Input: part model. Units: mm. Frame: model coordinates. A direction names the side the tool comes from. Round coordinates to 2 decimals unless told otherwise and drop trailing zeros. Loops run counter-clockwise (first coordinate to the right, second up) from the corner with the lowest first, then second, coordinate; pieces in that order, holes last. Notation, with made-up numbers: (55.5, 77) -> (61.5, 77) arc R33 ccw to (61.5, 107) -> close; hole circle Ø7 at (34.5, -5). An arc over 180 degrees is marked (long way). Answer as a JSON object with one key per item and string values.
```python
from build123d import *

# Parameters (mm, degrees)
SKETCH1_R           = 8.8
SKETCH1_R_2         = 3
BOSS_EXTRUDE1_DEPTH = 19.5
SKETCH2_OUTSIDE_W   = 25.924
SKETCH2_OUTSIDE_H   = 25.924
SKETCH2_OUTSIDE_R   = 4.5
CUT_EXTRUDE1_DEPTH  = 6.5
SKETCH3_OUTSIDE_W   = 25.924
SKETCH3_OUTSIDE_H   = 25.924
SKETCH3_OUTSIDE_R   = 6.8
CUT_EXTRUDE2_DEPTH  = 11
SKETCH5_OUTSIDE_W   = 25.924
SKETCH5_OUTSIDE_H   = 25.924
SKETCH5_OUTSIDE_R   = 4.8
CUT_EXTRUDE3_DEPTH  = 7.5
CUT_EXTRUDE4_START  = -1
SKETCH4_OUTSIDE_W   = 25.924
SKETCH4_OUTSIDE_H   = 25.924
SKETCH4_OUTSIDE_R   = 6
CUT_EXTRUDE4_DEPTH  = 1
CUT_EXTRUDE5_START  = -1
SKETCH6_OUTSIDE_W   = 25.924
SKETCH6_OUTSIDE_H   = 25.924
SKETCH6_OUTSIDE_R   = 4
CUT_EXTRUDE5_DEPTH  = 1
CUT_EXTRUDE6_START  = -3
SKETCH6_2_OUTSIDE_W = 25.924
SKETCH6_2_OUTSIDE_H = 25.924
SKETCH6_2_OUTSIDE_R = 4
CUT_EXTRUDE6_DEPTH  = 2
CHAMFER1_SIZE       = 0.5


with BuildPart() as part:
    # Sketch1 → Boss-Extrude1 (new body)
    with BuildSketch(Plane.XY):
        Circle(SKETCH1_R)
        Circle(SKETCH1_R_2, mode=Mode.SUBTRACT)
    extrude(amount=BOSS_EXTRUDE1_DEPTH)

    # Sketch2 outside → Cut-Extrude1 (cut)
    with BuildSketch(Plane.XY.offset(19.5)):
        Rectangle(SKETCH2_OUTSIDE_W, SKETCH2_OUTSIDE_H)
        Circle(SKETCH2_OUTSIDE_R, mode=Mode.SUBTRACT)
    extrude(amount=-CUT_EXTRUDE1_DEPTH, mode=Mode.SUBTRACT)

    # Sketch3 outside → Cut-Extrude2 (cut)
    with BuildSketch(Plane(origin=(0, 0, 0), x_dir=(-1, 0, 0), z_dir=(0, 0, -1))):
        Rectangle(SKETCH3_OUTSIDE_W, SKETCH3_OUTSIDE_H)
        Circle(SKETCH3_OUTSIDE_R, mode=Mode.SUBTRACT)
    extrude(amount=-CUT_EXTRUDE2_DEPTH, mode=Mode.SUBTRACT)

    # Sketch5 outside → Cut-Extrude3 (cut)
    with BuildSketch(Plane(origin=(0, 0, 0), x_dir=(-1, 0, 0), z_dir=(0, 0, -1))):
        Rectangle(SKETCH5_OUTSIDE_W, SKETCH5_OUTSIDE_H)
        Circle(SKETCH5_OUTSIDE_R, mode=Mode.SUBTRACT)
    extrude(amount=-CUT_EXTRUDE3_DEPTH, mode=Mode.SUBTRACT)

    # Sketch4 outside → Cut-Extrude4 (cut)
    with BuildSketch(Plane(origin=(0, 0, 7.5), x_dir=(-1, 0, 0), z_dir=(0, 0, -1)).offset(CUT_EXTRUDE4_START)):
        Rectangle(SKETCH4_OUTSIDE_W, SKETCH4_OUTSIDE_H)
        Circle(SKETCH4_OUTSIDE_R, mode=Mode.SUBTRACT)
    extrude(amount=-CUT_EXTRUDE4_DEPTH, mode=Mode.SUBTRACT)

    # Sketch6 outside → Cut-Extrude5 (cut)
    with BuildSketch(Plane(origin=(0, 0, 0), x_dir=(-1, 0, 0), z_dir=(0, 0, -1)).offset(CUT_EXTRUDE5_START)):
        Rectangle(SKETCH6_OUTSIDE_W, SKETCH6_OUTSIDE_H)
        Circle(SKETCH6_OUTSIDE_R, mode=Mode.SUBTRACT)
    extrude(amount=-CUT_EXTRUDE5_DEPTH, mode=Mode.SUBTRACT)

    # Sketch6<2> outside → Cut-Extrude6 (cut)
    with BuildSketch(Plane(origin=(0, 0, 0), x_dir=(-1, 0, 0), z_dir=(0, 0, -1)).offset(CUT_EXTRUDE6_START)):
        Rectangle(SKETCH6_2_OUTSIDE_W, SKETCH6_2_OUTSIDE_H)
        Circle(SKETCH6_2_OUTSIDE_R, mode=Mode.SUBTRACT)
    extrude(amount=-CUT_EXTRUDE6_DEPTH, mode=Mode.SUBTRACT)

    # Chamfer1
    chamfer1_edges = [part.edges().sort_by_distance(p)[0] for p in [
        (-4.5, 0, 19.5),
    ]]
    chamfer(chamfer1_edges, length=CHAMFER1_SIZE)


solid = part.part
```
1) Contact query for flat-ended pins moving along their axis: P1, Ø1.5, axis at y = 3, z = 9.5, coming from the -X side; P2, Ø5, axis at y = -5.5, z = 11, coming from the +X side; P3, Ø2, axis at y = -4, z = 3, coming from the -X side. Output: stop coordinate, or through.
Output:
{"P1": "stops at x = -6.42", "P2": "stops at x = 8.27", "P3": "stops at x = -3.75"}
2) Ray query, probe 1 along Y at (x, z) = (0, 4); probe 2 along Y at (x, z) = (0, 13.25); probe 3 along Z at (x, y) = (4, -1.75). Return the intervals inside material, ascending.
Output:
{"probe 1": "y = -4 to -3, 3 to 4", "probe 2": "y = -4.5 to -3, 3 to 4.5", "probe 3": "z = 0 to 1, 2 to 3, 5 to 19.13"}
3) Reachability of faces 1 (the face through (1, 3, 19.5)), 2 (the face through (-2.58, 4.05, 0.49)), 3 (the face through (-0.59, 4.46, 16.04)), 4 (the face through (1, -3, 0)), 5 (the face through (2, 4, 1)) from +Z, -Z, +X, -X, +Y, -Y: full face, straight path, thin tool, end or side. Return the list, or none.
Output:
{"face 1": "+Z, +X, -X, +Y, -Y", "face 2": "-Z", "face 3": "+Z", "face 4": "-Z, +X, -X, +Y, -Y", "face 5": "none"}
4) Section B-B, the plane z = 18. Output: boundary loops of the cut face in (x, y), plus the area to 3 significant figures.
Output:
{"outline": "circle Ø9 at (0, 0); hole circle Ø6 at (0, 0)", "area": "35.3 mm^2"}
5) Draft query along Z for faces 6 (the face through (8.394, 2.643, 11.986)), 7 (the face through (6, 0, 9)), 8 (the face through (4, -4, 13)). Return one class per face: +Z half, -Z half, draft (parallel to the pull), parting line (faces both ways), or undercut.
Output:
{"face 6": "draft", "face 7": "undercut", "face 8": "+Z half"}
6) Section A-A, the plane z = 7. Output: boundary loops of the cut face in (x, y).
Output:
{"outline": "circle Ø9.6 at (0, 0); hole circle Ø6 at (0, 0)"}
